Autodesk Inventor part; units mm, degrees
ref_plane "YZ Plane" through (0, 0, 0) normal (1, 0, 0) x (0, 1, 0)
ref_plane "XZ Plane" through (0, 0, 0) normal (0, 1, 0) x (-1, 0, 0)
ref_plane "XY Plane" through (0, 0, 0) normal (0, 0, 1) x (1, 0, 0)
sketch "Sketch1" plane through (0, 0, 0) normal (0, 0, 1) x (1, 0, 0)
  line L0 (0, 0) -> (85, 0)
  line L1 (85, 0) -> (85, 60)
  line L2 (85, 60) -> (0, 60)
  line L3 (0, 60) -> (0, 0)
  line L4 (0, 60) -> (35, 60)
  line L5 (35, 60) -> (35, 70)
  line L6 (35, 70) -> (55, 70)
  line L7 (55, 70) -> (85, 60)
  line L8 (35, 70) -> (0, 60)
  dimension "d0" = 85
  dimension "d1" = 60
  dimension "d2" = 35
  dimension "d3" = 10
  dimension "d4" = 20
extrude "Extrusion1" add sketch "Sketch1" along normal blind 60
fillet "Fillet1" radius 8 2 edges at (85, 0, 30) (0, 0, 30)
fillet "Fillet2" radius 2 16 edges at (82.6569, 2.3431, 60) (42.5, 0, 60) (2.3431, 2.3431, 60) (0, 34, 60) (85, 34, 60) (70, 65, 60) (45, 70, 60) (17.5, 65, 60) (82.6569, 2.3431, 0) (42.5, 0, 0) (2.3431, 2.3431, 0) (0, 34, 0) (85, 34, 0) (70, 65, 0) (45, 70, 0) (17.5, 65, 0)
sketch "Sketch2" plane through (0, 0, 0) normal (0, 0, -1) x (-1, 0, 0)
  point P0 (0, 0)
sketch "Sketch3" plane through (0, 0, 0) normal (0, 0, -1) x (-1, 0, 0)
  line L0 (-85, 8) -> (-85, 60)
  circle A0 centre (-27.9194, 43) radius 7.5
  circle A1 centre (-56.1406, 43) radius 7.5
  point P0 (0, 0)
  dimension "d12" = 15
extrude "Extrusion2" cut sketch "Sketch3" against normal blind 5
properties part number "SCALE HEAD"
Model file for the job. Use its own axes, mm. A direction names the side the tool comes from. Coordinates: 2 decimals unless noted, no trailing zeros. Order: outer loops, then holes, each group sorted by start corner. A loop starts at its lowest first (then second) coordinate and runs counter-clockwise, first axis right, second up. Notation, with made-up numbers: (82.5, -22) - (90.5, -22) arc R6 cw to (90.5, -12) - close; hole circle Ø7 at (76, 36). An arc over 180 degrees is marked (long way). Return JSON: item names as keys, results as strings. Group by question number.
1) Probe line 1 (Y direction, x = 8, z = 41); line 2 (Y direction, x = 78.5, z = 28); line 3 (Z direction, x = 14.5, y = 62.5). List the from-to ranges inside material, lowest first. Write a range as from..to.
2) Mould opens along Y. For faces 3 (the cylindrical face through (70, 64.4, 0.6)), 4 (the cylindrical face through (0.6, 33.64, 59.43)), 5 (the flat face through (28, 43, 5)) say: released by +Y, released by -Y, zero draft, split by the parting line, or undercut.
3) Saw through at B-B, the plane y = 43. Write the cut outline in (x, z).
4) Saw through at A-A, the plane z = 38.5. Write the cut outline in (x, y).
5) Flat gauge pin, fed straight in: P1, Ø7.5, axis at x = 57, y = 40, coming from the -Z side. Where does the tip first touch, or does it go through?
6) Tool access for faces 1 (the cylindrical face through (24.459, 36.346, 2.465)), 2 (the flat face through (42, 35, 60)): list every direction of +Z, -Z, +X, -X, +Y, -Y with a clear straight run to the whole face (end or side of a thin tool).
Values found:
{
 "1": {"line 1": "y = 0..62.29", "line 2": "y = 0.14..62.17", "line 3": "z = 0.04..59.96"},
 "2": {"face 3": "released by +Y", "face 4": "zero draft", "face 5": "undercut"},
 "3": {"outline": "(0, 2) arc R2 ccw to (2, 0) - (20.42, 0) - (20.42, 5) - (35.42, 5) - (35.42, 0) - (48.64, 0) - (48.64, 5) - (63.64, 5) - (63.64, 0) - (83, 0) arc R2 ccw to (85, 2) - (85, 58) arc R2 ccw to (83, 60) - (2, 60) arc R2 ccw to (0, 58) - close"},
 "4": {"outline": "(0, 8) arc R8 ccw to (8, 0) - (77, 0) arc R8 ccw to (85, 8) - (85, 60) - (55, 70) - (35, 70) - (0, 60) - close"},
 "5": {"P1": "stops at z = 5"},
 "6": {"face 1": "-Z", "face 2": "+Z, +X, -X, +Y, -Y"}
}
